from build123d import *

# Parameters (mm, degrees)
ESQUISSE2_W             = 200
ESQUISSE2_H             = 450
BOSS_EXTRU_1_DEPTH      = 110
ESQUISSE3_W             = 193.65
ESQUISSE3_H             = 443.65
ENL_V_MAT_EXTRU_1_DEPTH = 108
ESQUISSE5_W             = 107.95
ESQUISSE5_H             = 175.55
BOSS_EXTRU_2_DEPTH      = 38.1
ESQUISSE4_W             = 101.6
ESQUISSE4_H             = 169.2
ENL_V_MAT_EXTRU_2_DEPTH = 41.275


with BuildPart() as part:
    # Esquisse2 → Boss.-Extru.1 (new, symmetric)
    with BuildSketch(Plane.XY):
        Rectangle(ESQUISSE2_W, ESQUISSE2_H)
    extrude(amount=BOSS_EXTRU_1_DEPTH, both=True)

    # Esquisse3 → Enlèv. mat.-Extru.1 (cut, symmetric)
    with BuildSketch(Plane.XY):
        Rectangle(ESQUISSE3_W, ESQUISSE3_H)
    extrude(amount=ENL_V_MAT_EXTRU_1_DEPTH, both=True, mode=Mode.SUBTRACT)

    # Esquisse5 → Boss.-Extru.2 (add)
    with BuildSketch(Plane(origin=(0, 225, 0), x_dir=(1, 0, 0), z_dir=(0, 1, 0))):
        with Locations((23.8, 0)):
            Rectangle(ESQUISSE5_W, ESQUISSE5_H)
    extrude(amount=BOSS_EXTRU_2_DEPTH)

    # Esquisse4 → Enlèv. mat.-Extru.2 (cut)
    with BuildSketch(Plane(origin=(0, 263.1, 0), x_dir=(1, 0, 0), z_dir=(0, 1, 0))):
        with Locations((23.8, 0)):
            Rectangle(ESQUISSE4_W, ESQUISSE4_H)
    extrude(amount=-ENL_V_MAT_EXTRU_2_DEPTH, mode=Mode.SUBTRACT)


solid = part.part
CAD build for the part. Positions are in the model's coordinates, mm. A direction names the side the tool comes from. Coordinates: 2 decimals unless noted, no trailing zeros. Loops run counter-clockwise (first coordinate to the right, second up) from the corner with the lowest first, then second, coordinate; pieces in that order, holes last. Notation, with made-up numbers: (34.25, 60) - (61.25, 60) arc R13 cw to (61.25, 72) - close; hole circle Ø10 at (22, 15). An arc over 180 degrees is marked (long way). Write item = value, one per line. Start each with the question number.
Q1. Drill centre lines: L1, parallel to X at y = 159, z = -36.5 (3 decimals); L2, parallel to Z at x = -68, y = -183; L3, parallel to Y at x = 44, z = 93 (3 decimals). Where is each one in solid material? Low to high.
Q2. Cut at A-A, the plane x = -59.5. List the corners of the cut face in (y, z) (3 decimals).
Q3. Cut at D-D, the plane z = -45.5. List the corners of the cut face in (x, y) (3 decimals).
Q4. Flat gauge pins, fed straight in: pin 1 Ø12.5 at (y, z) = (239, -32.5) entering from +X (3 decimals); pin 2 Ø20.5 at (x, y) = (1.5, 238.5) entering from +Z (3 decimals); pin 3 Ø20.5 at (y, z) = (243.5, -35.5) entering from -X (3 decimals). Where does each tip first touch, or does it go through?
Q5. Cut at B-B, the plane y = -150.5. List the corners of the cut face in (x, z) (3 decimals), then the cut area to 3 significant figures.
Q6. Cut at C-C, the plane x = -21. List the corners of the cut face in (y, z) (3 decimals).
Q7. Which spindle directions (+Z, -Z, +X, -X, +Y, -Y) get a long thin tool onto all of the face, cutting with end or side? Do faces 5 (the flat face through (23, 243, -84.6)), 6 (the flat face through (-96.825, -3, 2)), 7 (the flat face through (-30.175, 244, 1)). Say none if no direction does.
Q8. Pull direction Y, two halves, no side cores. Call faces 1 (the flat face through (-1, -221.825, 2)), 2 (the flat face through (-1, -225, 2)), 3 (the flat face through (-1, 3, 108)), 4 (the flat face through (100, -3, 2)): pulls with the +Y half, pulls with the -Y half, needs draft (parallel to the pull), parting line crosses it, or undercut.
Computed:
q1.L1 = -100 to -96.825, 96.825 to 100
q1.L2 = -110 to -108, 108 to 110
q1.L3 = -225 to -221.825, 221.825 to 225
q2.outline = (-225, -110) - (225, -110) - (225, 110) - (-225, 110) - close; hole (-221.825, -108) - (221.825, -108) - (221.825, 108) - (-221.825, 108) - close
q3.outline = (-100, -225) - (100, -225) - (100, 225) - (77.775, 225) - (77.775, 263.1) - (74.6, 263.1) - (74.6, 221.825) - (96.825, 221.825) - (96.825, -221.825) - (-96.825, -221.825) - (-96.825, 221.825) - (-27, 221.825) - (-27, 263.1) - (-30.175, 263.1) - (-30.175, 225) - (-100, 225) - close
q4.pin_1 = 77.775
q4.pin_2 = 87.775
q4.pin_3 = -30.175
q5.outline = (-100, -110) - (100, -110) - (100, 110) - (-100, 110) - close; hole (-96.825, -108) - (96.825, -108) - (96.825, 108) - (-96.825, 108) - close
q5.area = 2,170 mm²
q6.outline = (-225, -110) - (225, -110) - (225, -87.775) - (263.1, -87.775) - (263.1, -84.6) - (221.825, -84.6) - (221.825, -108) - (-221.825, -108) - (-221.825, 108) - (221.825, 108) - (221.825, 84.6) - (263.1, 84.6) - (263.1, 87.775) - (225, 87.775) - (225, 110) - (-225, 110) - close
q7.face_5 = +Y
q7.face_6 = none
q7.face_7 = +Z, -Z, -X, +Y
q8.face_1 = undercut
q8.face_2 = pulls with the -Y half
q8.face_3 = undercut
q8.face_4 = needs draft
